Source: CAD feature listing. Evaluate the final solid. Frame: model axes, mm. Face numbers are marked on the shaded views. A direction names the side the tool comes from. Round coordinates to 2 decimals unless told otherwise and drop trailing zeros. Order: outer loops, then holes, each group sorted by start corner. A loop starts at its lowest first (then second) coordinate and runs counter-clockwise, first axis right, second up. Notation, with made-up numbers: (-20.5, 45.25) - (20.5, 45.25) arc R19 ccw to (20.5, 71.25) - close; hole circle Ø6 at (67.5, 28). An arc over 180 degrees is marked (long way). Use one line per item in the form item = value. Start each with the question number.
Q1. Cut plane A-A, the plane y = 56.3. Return the cut outline in (x, z).
Q2. Set-up query: the marked faces 1, 2 and 3. Return all of +Z, -Z, +X, -X, +Y, -Y with unobstructed straight access to the full face (end or side cutting, diameter ignored); none if empty.
Q3. Cut plane B-B, the plane y = 65.5. Return the cut outline in (x, z).
Q4. Ray query, line 1 (Z direction, x = 24.5, y = 72); line 2 (X direction, y = 45.5, z = 42.5); line 3 (Y direction, x = 24, z = 40). Return the intervals inside material, ascending. Write a range as [from, to].
Q5. Draft query along X for the marked faces 4, 5 and 6. Return one class per face: released by +X, released by -X, zero draft, split by the parting line, or undercut.
Q6. Cut plane C-C, the plane x = 37.5. Return the cut outline in (y, z), and give its area (3 significant figures).
Q7. Pin query (flat end, axial travel): pin 1 Ø3.5 at (x, z) = (29.5, 19.5) entering from -Y; pin 2 Ø3 at (x, z) = (39, 28.5) entering from +Y; pin 3 Ø3 at (x, y) = (54, 46) entering from -Z. Return the tip coordinate at first contact, or that it passes through.
Q8. Cut plane D-D, the plane z = 40. Give the number of separate pieces and of enclosed holes in the cut face, and give its area (3 significant figures).
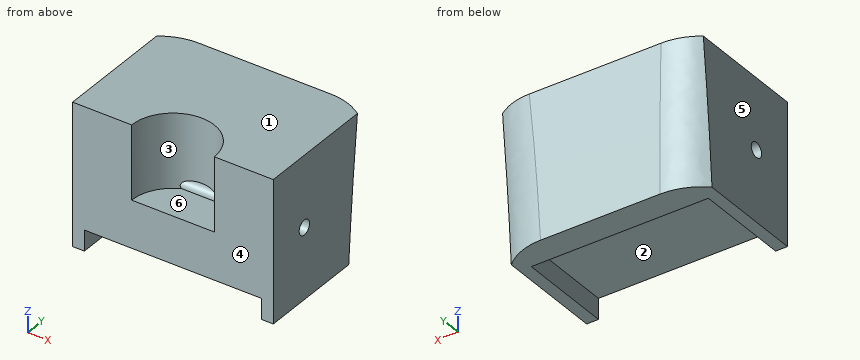
Autodesk Inventor part; units mm, degrees
ref_plane "YZ Plane" through (0, 0, 0) normal (1, 0, 0) x (0, 1, 0)
ref_plane "XZ Plane" through (0, 0, 0) normal (0, 1, 0) x (-1, 0, 0)
ref_plane "XY Plane" through (0, 0, 0) normal (0, 0, 1) x (1, 0, 0)
sketch "Sketch1" plane through (0, 0, 0) normal (0, 0, 1) x (1, 0, 0)
  line L0 (0, 0) -> (80, 0)
  line L1 (80, 0) -> (80, 82.6)
  line L2 (80, 82.6) -> (0, 82.6)
  line L3 (0, 82.6) -> (0, 0)
  dimension "d0" = 80
  dimension "d1" = 82.6
extrude "Extrusion1" add sketch "Sketch1" along normal blind 162.5
sketch "Sketch2" plane through (0, 82.6, 0) normal (0, 1, 0) x (1, 0, 0)
  line L0 (0, -162.5) -> (80, -162.5)
  line L1 (-12.5, -162.5) -> (0, -162.5)
  line L2 (80, -162.5) -> (92.5, -162.5)
  line L3 (0, 0) -> (80, 0)
  line L4 (0, 0) -> (0, -162.5)
  line L5 (80, 0) -> (80, -162.5)
  arc A0 (-12.5, -162.5) -> (0, 0) centre (-1199.9534, 10.5733) ccw
  arc A1 (80, 0) -> (92.5, -162.5) centre (1279.9534, 10.5733) ccw
  dimension "d4" = 12.5
  dimension "d5" = 12.5
  dimension "d19" = 1200
  dimension "d20" = 1200
extrude "Extrusion2" add sketch "Sketch2" against normal blind 82.6 contours L1 A0 L4 | L5 A1 L2
sketch "Sketch4" plane through (0, 0, 0) normal (0, 0, -1) x (-1, 0, 0)
  circle A0 centre (-17.4, 59.41) radius 2.5
  circle A1 centre (-62.6, 59.41) radius 2.5
  circle A2 centre (-62.6, 23.19) radius 2.5
  circle A3 centre (-17.4, 23.19) radius 2.5
  line L0 (-80, 82.6) -> (0, 82.6)
  line L1 (-17.4, 23.19) -> (-62.6, 23.19) construction
  line L2 (-62.6, 23.19) -> (-62.6, 59.41) construction
  line L3 (-80, 0) -> (-80, 82.6)
  point P0 (0, 0)
  point P1 (-60.8187, 82.6)
  point P2 (-19.1813, 82.6)
  point P3 (-40, 23.19)
  point P4 (-40, 82.6)
  dimension "d10" = 5
  dimension "d11" = 5
  dimension "d12" = 5
  dimension "d13" = 5
  dimension "d14" = 23.19
  dimension "d15" = 45.2
  dimension "d16" = 36.22
extrude "Extrusion3" cut sketch "Sketch4" against normal blind 25
sketch "Sketch5" plane through (0, 0, 0) normal (0, 0, -1) x (-1, 0, 0)
  line L0 (12.5, 0) -> (-92.5, 0)
  line L1 (-92.5, 0) -> (-92.5, 41.3)
  line L2 (-92.5, 41.3) -> (12.5, 41.3)
  line L3 (12.5, 41.3) -> (12.5, 0)
  point P0 (0, 0)
  point P1 (12.5, 20)
  point P2 (-92.5, 20)
  dimension "d22" = 41.3
extrude "Extrusion4" cut sketch "Sketch5" against normal through all
sketch "Sketch6" plane through (0, 41.3, 0) normal (0, -1, 0) x (1, 0, 0)
  line L0 (75, 15) -> (5, 15)
  line L1 (5, 15) -> (5, 65)
  line L2 (5, 65) -> (75, 65)
  line L3 (75, 65) -> (75, 15)
  line L4 (80, 0) -> (0, 0)
  point P0 (40, 15)
  point P1 (40, 0)
  dimension "d25" = 70
  dimension "d26" = 50
  dimension "d27" = 15
extrude "Extrusion5" cut sketch "Sketch6" against normal blind 32.5
sketch "Sketch8" plane through (0, 0, 0) normal (1, 0, 0) x (0, 1, 0)
  line L0 (82.6, 162.5) -> (93.8, 162.5)
  line L1 (41.3, 162.5) -> (41.3, 0)
  line L2 (82.6, 0) -> (41.3, 0)
  arc A0 (93.8, 162.5) -> (82.6, 0) centre (2580.9593, -90.5586) ccw
  line L3 (82.6, 162.5) -> (41.3, 162.5)
  line L4 (82.6, 162.5) -> (82.6, 0)
  point P0 (0, 0)
  dimension "d32" = 2500
  dimension "d38" = 11.2
extrude "Extrusion6" add sketch "Sketch8" along normal blind 93 and the other way blind 13 contours L0 A0 L4
sketch "Sketch13" plane through (-13, 82.6, 0) normal (0, -1, 0) x (1, 0, 0)
  arc A0 (13, 0) -> (0.5, 162.5) centre (-1186.9534, -10.5733) ccw
  line L0 (0, 162.5) -> (0.5, 162.5)
  line L1 (0, 0) -> (0, 162.5)
  line L2 (13, 0) -> (0, 0)
  arc A1 (105.5, 162.5) -> (93, 0) centre (1292.9534, -10.5733) ccw
  line L3 (106, 0) -> (93, 0)
  line L4 (106, 162.5) -> (106, 0)
  line L5 (105.5, 162.5) -> (106, 162.5)
  point P0 (13, 0)
extrude "Extrusion9" cut sketch "Sketch13" against normal through all
fillet "Fillet4" radius 20 2 edges at (-3.5176, 86.9111, 81.8462) (83.5176, 86.9111, 81.8462)
sketch "Sketch34" plane through (0, 41.3, 0) normal (0, -1, 0) x (1, 0, 0)
  line L0 (75, 65) -> (75, 15)
  line L1 (75, 15) -> (5, 15)
  line L2 (5, 15) -> (5, 65)
  line L3 (5, 65) -> (75, 65)
  arc A0 (0, 0) -> (-12.5, 162.5) centre (-1199.9534, -10.5733) ccw
  line L4 (80, 0) -> (0, 0)
  arc A1 (92.5, 162.5) -> (80, 0) centre (1279.9534, -10.5733) ccw
  line L5 (-12.5, 162.5) -> (92.5, 162.5)
  point P0 (0, 0)
extrude "Extrusion24" cut sketch "Sketch34" against normal through all
sketch "Sketch35" plane through (0, 73.8, 0) normal (0, -1, 0) x (1, 0, 0)
  line L0 (75, 15) -> (5, 15)
  line L1 (75, 65) -> (75, 15)
  line L2 (5, 65) -> (75, 65)
  line L3 (5, 15) -> (5, 65)
  point P0 (0, 0)
extrude "Extrusion25" add sketch "Sketch35" along normal blind 32.5
sketch "Sketch36" plane through (0, 41.3, 0) normal (0, -1, 0) x (1, 0, 0)
  line L0 (10, 15) -> (70, 15)
  line L1 (70, 15) -> (70, 23)
  line L2 (70, 23) -> (10, 23)
  line L3 (10, 23) -> (10, 15)
  line L4 (5, 15) -> (75, 15)
  point P0 (0, 0)
  point P1 (40, 23)
  point P2 (40, 15)
  point P3 (40, 15)
  dimension "d112" = 8
  dimension "d113" = 60
extrude "Extrusion26" cut sketch "Sketch36" against normal blind 32.5
sketch "Sketch37" plane through (5, 41.3, 65) normal (-1, 0, 0) x (0, 0, 1)
  circle A0 centre (-25, 15) radius 2.5
  line L0 (0, 0) -> (-50, 0)
  point P0 (-65, -41.3)
  point P1 (-25, 0)
  dimension "d116" = 5
  dimension "d117" = 15
extrude "Extrusion27" cut sketch "Sketch37" against normal through all
sketch "Sketch38" plane through (0, 41.3, 0) normal (0, -1, 0) x (1, 0, 0)
  line L0 (75, 15) -> (5, 15)
  line L1 (5, 15) -> (5, 65)
  line L2 (5, 65) -> (75, 65)
  line L3 (75, 65) -> (75, 15)
  line L4 (75, 65) -> (5, 65)
  line L5 (75, 15) -> (75, 65)
  line L6 (74, 16) -> (6, 16)
  line L7 (6, 16) -> (6, 64)
  line L8 (6, 64) -> (74, 64)
  line L9 (74, 64) -> (74, 16)
  point P0 (0, 0)
  dimension "d120" = 1
extrude "Extrusion28" cut sketch "Sketch38" against normal through all
sketch "Sketch39" plane through (6, 41.3, 64) normal (0, 0, 1) x (1, 0, 0)
  line L0 (68, 0) -> (0, 0)
  line L1 (4, 0) -> (64, 0)
  circle A0 centre (34, 0) radius 14
  point P0 (-6, -41.3)
  dimension "d123" = 28
extrude "Extrusion29" cut sketch "Sketch39" against normal blind 25
equation "\"d5\" = d4"
properties part number "AA008" material "ABS Plastic"
Completed:
q1.outline = (6, 16) - (10, 16) - (10, 23) - (70, 23) - (70, 16) - (74, 16) - (74, 37.5) - (6, 37.5) - close; (6, 42.5) - (74, 42.5) - (74, 64) - (6, 64) - close
q2.face_1 = +Z, +X, -X, +Y, -Y
q2.face_2 = -Z, -Y
q2.face_3 = +Z, -Y
q3.outline = (6, 16) - (10, 16) - (10, 23) - (70, 23) - (70, 16) - (74, 16) - (74, 64) - (6, 64) - close
q4.line_1 = [23, 64]
q4.line_2 = [6, 26.64], [53.36, 74]
q4.line_3 = [41.3, 53.8], [58.8, 84.37]
q5.face_4 = zero draft
q5.face_5 = released by -X
q5.face_6 = undercut
q6.outline = (41.3, 23) - (73.8, 23) - (73.8, 16) - (83.23, 16) arc R2500 cw to (85.74, 64) - (55.07, 64) - (55.07, 42.18) arc R2.5 cw (long way) to (54.01, 39) - (41.3, 39) - close
q6.area = 1,480 mm2
q7.pin_1 = 73.8
q7.pin_2 = 83.87
q7.pin_3 = 23
q8.separate_pieces = 3
q8.enclosed_holes = 0
q8.area = 2,250 mm2
